Source: CAD feature listing. Evaluate the final solid. Frame: model axes, mm. Face numbers are marked on the shaded views. A direction names the side the tool comes from. Coordinates: 2 decimals unless noted, no trailing zeros. Loops run counter-clockwise (first coordinate to the right, second up) from the corner with the lowest first, then second, coordinate; pieces in that order, holes last.
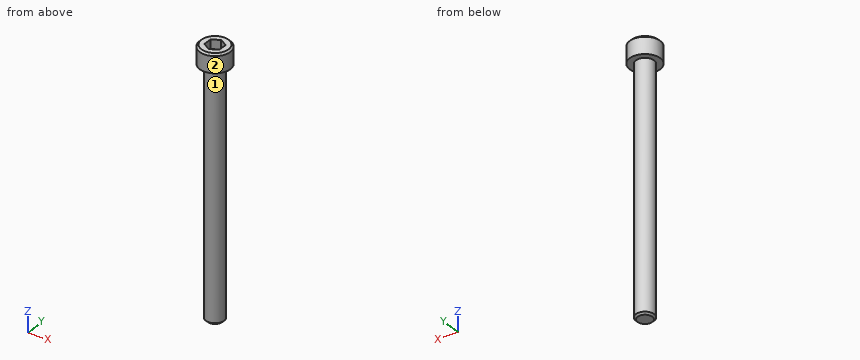
Autodesk Inventor part; units mm, degrees
ref_plane "YZ Plane" through (0, 0, 0) normal (1, 0, 0) x (0, 1, 0)
ref_plane "XZ Plane" through (0, 0, 0) normal (0, 1, 0) x (-1, 0, 0)
ref_plane "XY Plane" through (0, 0, 0) normal (0, 0, 1) x (1, 0, 0)
sketch "Sketch1" plane through (0, 0, 0) normal (0, 0, 1) x (1, 0, 0)
  circle A0 centre (0, 0) radius 3
  dimension "Diameter" = 6
extrude "Extrusion1" add sketch "Sketch1" along normal blind 80
sketch "Sketch2" plane through (0, 0, 80) normal (0, 0, 1) x (1, 0, 0)
  circle A0 centre (0, 0) radius 3
  circle A1 centre (0, 0) radius 5
  dimension "Head_Diameter" = 10
extrude "Extrusion2" add sketch "Sketch2" along normal blind 6 contours A0 | A1
sketch "Sketch3" plane through (0, 0, 86) normal (0, 0, 1) x (1, 0, 0)
  circle A0 centre (0, 0) radius 5
  circle A1 centre (0, 0) radius 2.8868 construction
  line L0 (0, 2.8868) -> (2.5, 1.4434)
  line L1 (2.5, -1.4434) -> (2.5, 1.4434)
  line L2 (0, 2.8868) -> (-2.5, 1.4434)
  line L3 (-2.5, -1.4434) -> (-2.5, 1.4434)
  line L4 (-2.5, -1.4434) -> (0, -2.8868)
  line L5 (2.5, -1.4434) -> (0, -2.8868)
  dimension "Hex_Width" = 5
extrude "Extrusion3" cut sketch "Sketch3" against normal blind 3 contours L0 L1 L5 L4 L3 L2
thread "Thread1"
chamfer "Chamfer1" distance 0.6 angle 45 2 edges at (-5, 0, 86) (-3, 0, 0)
equation "\"d9\" = ThreadLength"
equation "\"d12\" = Chamfer"
equation "\"ThreadLength\" = 24"
properties part number "SCREW, SOCKET HD, P, 12.9, M6X1X80MM"
Q1. Section query B-B on z = 65.5. Return the cut outline in (x, y).
Q2. Section query A-A on y = 0. Return the cut outline in (x, z).
Q3. Material intervals for line 1 along Z through (x, y) = (4.25, -0.25); line 2 along Z through (x, y) = (-1.25, -1.75); line 3 along X through (y, z) = (-0.75, 39.5), sorted ascending.
Q4. First-contact query: pin 1 Ø1.5 at (x, z) = (1, 65.5) entering from +Y; pin 2 Ø2 at (y, z) = (1.5, 47.5) entering from +X; pin 3 Ø1.5 at (x, y) = (0, -1) entering from +Z. Flat tips, straight axial feed; report the tip coordinate or a pass-through.
Q5. Reachability of the marked faces 1 and 2 from +Z, -Z, +X, -X, +Y, -Y: full face, straight path, thin tool, end or side. Return the list, or none.
Resolved:
1. outline: circle Ø6 at (0, 0)
2. outline: (-5, 80) - (-3, 80) - (-3, 0.6) - (-2.4, 0) - (2.4, 0) - (3, 0.6) - (3, 80) - (5, 80) - (5, 85.4) - (4.4, 86) - (2.5, 86) - (2.5, 83) - (-2.5, 83) - (-2.5, 86) - (-4.4, 86) - (-5, 85.4) - close
3. line 1: z = 80 to 86
3. line 2: z = 0 to 83
3. line 3: x = -2.9 to 2.9
4. pin 1: stops at y = 2.99
4. pin 2: stops at x = 2.96
4. pin 3: stops at z = 83
5. face 1: -Z
5. face 2: +Z, -Z
